Geometry check sheet. Reference: the model listing, model coordinates, mm. A direction names the side the tool comes from. Give positions to 0.01 mm unless a question says otherwise; leave off trailing zeros. Order: outer loops, then holes, each group sorted by start corner. A loop starts at its lowest first (then second) coordinate and runs counter-clockwise, first axis right, second up. Notation, with made-up numbers: M 28.5,-9 L 38.5,-9 A7 cw 38.5,2 Z; hole C 19.25,86 d6. An arc over 180 degrees is marked long. Put each result on its own line as item: value. Start each with the question number.
Q1. Access from +Z, -Z, +X, -X, +Y, -Y to the whole of each face (thin tool, end or side, straight path). Record for faces 5 (the flat face through (0.661, 0, 34)), 6 (the flat face through (0, 4, 8)), 7 (the flat face through (-3, 4, 29.595)).
Q2. Section check D-D on x = 10.5. Record the cut outline in (y, z).
Q3. Material ranges on L1, parallel to Y at x = -0.5, z = 34; L2, parallel to Y at x = 10.8, z = 0; L3, parallel to Z at x = -4, y = 6.75, recorded low to high.
Q4. Section check C-C on x = 1.5. Record the cut outline in (y, z), then the cut area to 3 significant figures.
Q5. Mould release check, pull along Y, two halves, no side actions. Record for faces 1 (the cylindrical face through (12, 2, 0)), 2 (the cylindrical face through (0.059, 4.049, 29.024)), 3 (the flat face through (2, 0, 9)), 4 (the cylindrical face through (-2.46, -1.719, 40.886)): +Y half, -Y half, draft (parallel to the pull), parting line (faces both ways), or undercut.
Q6. Go/stop test with flat-tipped pins: pin 1 (4 mm diameter, centred on y = 3, z = 7, fed in from -X); pin 2 (8 mm diameter, centred on x = 0, z = 24, fed in from +Y); pin 3 (4 mm diameter, centred on x = -2.5, z = 3, fed in from -Y). Record where each tip stops, or that it passes through.
Q7. Section check A-A on y = 4. Record the cut outline in (x, z), then the cut area to 3 significant figures.
Q8. Section check B-B on z = 0. Record the cut outline in (x, y).
```python
from build123d import *

# Parameters (mm, degrees)
SKETCH1_R           = 4.5
BOSS_EXTRUDE1_DEPTH = 8
SKETCH2_R           = 4.75
BOSS_EXTRUDE2_DEPTH = 3
SKETCH3_R           = 2
CUT_EXTRUDE1_DEPTH  = 5
BOSS_EXTRUDE3_DEPTH = 8
SKETCH5_W           = 7
SKETCH5_H           = 16
BOSS_EXTRUDE4_DEPTH = 20
FILLET1_START       = -7
FILLET1_DEPTH       = 18
FILLET1_START_2     = -6.339273926
FILLET1_2_DEPTH     = 7
SKETCH6_W           = 7
SKETCH6_H           = 7
CUT_EXTRUDE2_DEPTH  = 17
FILLET2_R           = 3
SKETCH7_R           = 1.75
CUT_EXTRUDE3_DEPTH  = 52.215801422
FILLET3_R           = 2


with BuildPart() as part:
    # Sketch1 → Boss-Extrude1 (new body)
    with BuildSketch(Plane(origin=(0, 0, 0), x_dir=(1, 0, 0), z_dir=(0, 1, 0))):
        with BuildLine():
            Line((0, 6), (11, 6))
            Line((11, 6), (11, -6))
            Line((11, -6), (0, -6))
            ThreePointArc((0, -6), (-6, 0), (0, 6))
        make_face()
        with Locations(Location((0, 0, 0), (0, 0, 270))):
            Circle(SKETCH1_R, mode=Mode.SUBTRACT)
    extrude(amount=BOSS_EXTRUDE1_DEPTH)

    # Sketch2 → Boss-Extrude2 (add)
    with BuildSketch(Plane(origin=(11, 0, 0), x_dir=(0, 0, -1), z_dir=(1, 0, 0))):
        with Locations(Location((0, 4, 0), (0, 0, 122.636897504))):
            Circle(SKETCH2_R)
    extrude(amount=BOSS_EXTRUDE2_DEPTH)

    # Sketch3 → Cut-Extrude1 (cut)
    with BuildSketch(Plane(origin=(14, 0, 0), x_dir=(0, 0, -1), z_dir=(1, 0, 0))):
        with Locations((0, 4)):
            Circle(SKETCH3_R)
    extrude(amount=-CUT_EXTRUDE1_DEPTH, mode=Mode.SUBTRACT)

    # Sketch4 → Boss-Extrude3 (add)
    with BuildSketch(Plane(origin=(0, 0, 0), x_dir=(1, 0, 0), z_dir=(0, 1, 0))):
        Polygon((0, -6), (0, -9.448137361), (-6.339273926, -23.042754167), (-6.339273926, -26.594616806), (0.660726074, -26.594616806), (0.660726074, -24.594616806), (7, -11), (7, -6), align=None)
    extrude(amount=BOSS_EXTRUDE3_DEPTH)

    # Sketch5 → Boss-Extrude4 (add)
    with BuildSketch(Plane.XY.offset(26.594616806)):
        with Locations((-2.839273926, 4)):
            Rectangle(SKETCH5_W, SKETCH5_H)
    extrude(amount=BOSS_EXTRUDE4_DEPTH)

    # Fillet1: read off the stored shape, not the designer's step
    # Fillet1 outline → Fillet1 (cut)
    with BuildSketch(Plane.YZ.offset(FILLET1_START)):
        with BuildLine():
            Line((-4, 26.594616806), (-2, 26.594616806))
            ThreePointArc((-2, 26.594616806), (-3.414213563, 27.180403244), (-4, 28.594616806))
            Line((-4, 28.594616806), (-4, 26.594616806))
        make_face()
        with BuildLine():
            ThreePointArc((12, 28.594616806), (11.414213563, 27.180403244), (10, 26.594616806))
            Line((10, 26.594616806), (12, 26.594616806))
            Line((12, 26.594616806), (12, 28.594616806))
        make_face()
    extrude(amount=FILLET1_DEPTH, mode=Mode.SUBTRACT)

    # Fillet1 2 outline → Fillet1 2 (add)
    with BuildSketch(Plane.YZ.offset(FILLET1_START_2)):
        with BuildLine():
            ThreePointArc((-2, 26.594616806), (-0.585786438, 26.008830368), (0, 24.594616806))
            Line((0, 24.594616806), (0, 26.594616806))
            Line((0, 26.594616806), (-2, 26.594616806))
        make_face()
        with BuildLine():
            ThreePointArc((8, 24.594616806), (8.585786438, 26.008830368), (10, 26.594616806))
            Line((10, 26.594616806), (8, 26.594616806))
            Line((8, 26.594616806), (8, 24.594616806))
        make_face()
    extrude(amount=FILLET1_2_DEPTH)

    # Sketch6 → Cut-Extrude2 (cut)
    with BuildSketch(Plane.XY.offset(46.594616806)):
        with Locations((-2.839273926, 4)):
            Rectangle(SKETCH6_W, SKETCH6_H)
    extrude(amount=-CUT_EXTRUDE2_DEPTH, mode=Mode.SUBTRACT)

    # Fillet2
    fillet2_edges = [part.edges().sort_by_distance(p)[0] for p in [
        (0.660726074, -1.75, 46.594616806),
        (-6.339273926, 9.75, 46.594616806),
        (0.660726074, 9.75, 46.594616806),
        (-6.339273926, -1.75, 46.594616806),
    ]]
    fillet(fillet2_edges, radius=FILLET2_R)

    # Sketch7 → Cut-Extrude3 (cut, through all)
    with BuildSketch(Plane(origin=(0, 12, 0), x_dir=(1, 0, 0), z_dir=(0, 1, 0))):
        with Locations(Location((-2.839273926, -42.594616806, 0), (0, 0, 180))):
            Circle(SKETCH7_R)
    extrude(amount=-CUT_EXTRUDE3_DEPTH, mode=Mode.SUBTRACT)

    # Fillet3
    fillet3_edges = [part.edges().sort_by_distance(p)[0] for p in [
        (-6.339273926, 4, 29.594616806),
        (0.660726074, 4, 29.594616806),
    ]]
    fillet(fillet3_edges, radius=FILLET3_R)


solid = part.part
```
Results found:
1. face 5: +Z, +X, +Y, -Y
1. face 6: -X, +Y, -Y
1. face 7: +Z, +X, -X
2. outline: M 0,-6 L 8,-6 L 8,6 L 0,6 Z; hole C 4,0 d4
3. L1: y = -4 to 0.5, 7.5 to 12
3. L2: y = 0 to 2, 6 to 8
3. L3: z = -4.47 to -2.06, 2.06 to 4.47, 18.03 to 29.59
4. outline: M 0,-6 L 8,-6 L 8,-4.24 L 0,-4.24 Z; M 0,4.24 L 8,4.24 L 8,22.79 L 0,22.79 Z
4. area: 162 mm^2
5. face 1: undercut
5. face 2: undercut
5. face 3: -Y half
5. face 4: draft
6. pin 1: stops at x = -3.32
6. pin 2: stops at y = 11.91
6. pin 3: stops at y = 0
7. outline: M -6.34,23.04 L 0,9.45 L 0,6 A6 ccw 0,-6 L 11,-6 L 11,-4.75 L 14,-4.75 L 14,-2 L 9,-2 L 9,2 L 14,2 L 14,4.75 L 11,4.75 L 11,6 L 7,6 L 7,11 L 0.66,24.59 L 0.66,27.59 A2 ccw -1.34,29.59 L -4.34,29.59 A2 ccw -6.34,27.59 Z; hole C 0,0 d9
7. area: 307 mm^2
8. outline: M -6,0 L -4.5,0 L -4.5,8 L -6,8 Z; M 4.5,0 L 11,0 L 11,-0.75 L 14,-0.75 L 14,2 L 9,2 L 9,6 L 14,6 L 14,8.75 L 11,8.75 L 11,8 L 4.5,8 Z
